from build123d import *

# Parameters (mm, degrees)
SKETCH1_R                                           = 60
SKETCH1_R_2                                         = 16.2
BOSS_EXTRUDE1_DEPTH                                 = 7
CSK_FOR_M6_COUNTERSUNK_FLAT_HEAD_SCREW1_D           = 6.6
CSK_FOR_M6_COUNTERSUNK_FLAT_HEAD_SCREW1_CSINK_D     = 12.6
CSK_FOR_M6_COUNTERSUNK_FLAT_HEAD_SCREW1_CSINK_ANGLE = 90


with BuildPart() as part:
    # Sketch1 → Boss-Extrude1 (new body)
    with BuildSketch(Plane.XY):
        Circle(SKETCH1_R)
        Circle(SKETCH1_R_2, mode=Mode.SUBTRACT)
    extrude(amount=BOSS_EXTRUDE1_DEPTH)

    # CSK for M6 Countersunk Flat Head Screw1 (through all)
    with Locations(Plane.XY.offset(7)):
        with Locations((-37.123106012, 37.123106012), (0, 52.5), (37.123106012, 37.123106012), (52.5, 0), (37.123106012, -37.123106012), (0, -52.5), (-37.123106012, -37.123106012), (-52.5, 0)):
            CounterSinkHole(CSK_FOR_M6_COUNTERSUNK_FLAT_HEAD_SCREW1_D / 2, CSK_FOR_M6_COUNTERSUNK_FLAT_HEAD_SCREW1_CSINK_D / 2, counter_sink_angle=CSK_FOR_M6_COUNTERSUNK_FLAT_HEAD_SCREW1_CSINK_ANGLE)


solid = part.part
CAD build for the part. Positions are in the model's coordinates, mm. Coordinates: 2 decimals unless noted, no trailing zeros. Order: outer loops, then holes, each group sorted by start corner. A loop starts at its lowest first (then second) coordinate and runs counter-clockwise, first axis right, second up.
Item 1: Pin check, flat tips, straight feed: pin 1 Ø2 at (x, z) = (-27, 1.5) entering from -Y; pin 2 Ø4 at (x, z) = (13, 2.5) entering from +Y; pin 3 Ø8.5 at (x, y) = (0, 52.5) entering from +Z; pin 4 Ø6 at (x, y) = (-52.5, 0) entering from -Z. Stop position of each tip, or through.
Check sheet entries:
pin 1: stops at y = -54.07
pin 2: stops at y = 58.98
pin 3: stops at z = 4.95
pin 4: passes through
Item 2: Drill centre lines: L1, parallel to Y at x = 0, z = 3.5; L2, parallel to X at y = -36, z = 3; L3, parallel to X at y = 37, z = 2.25. Where is each one in solid material? Low to high.
Check sheet entries:
L1: y = -60 to -55.8, -49.2 to -16.2, 16.2 to 49.2, 55.8 to 60
L2: x = -48 to -40.23, -34.02 to 34.02, 40.23 to 48
L3: x = -47.23 to -40.42, -33.83 to 33.83, 40.42 to 47.23
Item 3: Band-saw the part on C-C on x = 52.5. List the corners of the cut face in (y, z).
Check sheet entries:
outline: (-29.05, 0) - (-3.3, 0) - (-3.3, 4) - (-6.3, 7) - (-29.05, 7) - close; (3.3, 0) - (29.05, 0) - (29.05, 7) - (6.3, 7) - (3.3, 4) - close
Item 4: Band-saw the part on A-A on y = 0. List the corners of the cut face in (x, z), plus the area to 3 significant figures.
Check sheet entries:
outline: (-60, 0) - (-55.8, 0) - (-55.8, 4) - (-58.8, 7) - (-60, 7) - close; (-49.2, 0) - (-16.2, 0) - (-16.2, 7) - (-46.2, 7) - (-49.2, 4) - close; (16.2, 0) - (49.2, 0) - (49.2, 4) - (46.2, 7) - (16.2, 7) - close; (55.8, 0) - (60, 0) - (60, 7) - (58.8, 7) - (55.8, 4) - close
area: 503 mm2
Item 5: Two-plate mould, pull along X, no slides. Class faces 1 (the face through (-59.94, 2.64, 3.45)), 2 (the face through (12, -12, 0)), 3 (the face through (49.21, 1.03, 4.15)): +X half, -X half, draft (parallel to the pull), parting line (faces both ways), or undercut.
Check sheet entries:
face 1: parting line
face 2: draft
face 3: undercut
